Here's the drawing with two shaded views (mm, measured from the low corner). I have some questions. Give positions to 0.01 mm unless a question says otherwise; leave off trailing zeros. Loops run counter-clockwise (first coordinate to the right, second up) from the corner with the lowest first, then second, coordinate; pieces in that order, holes last.
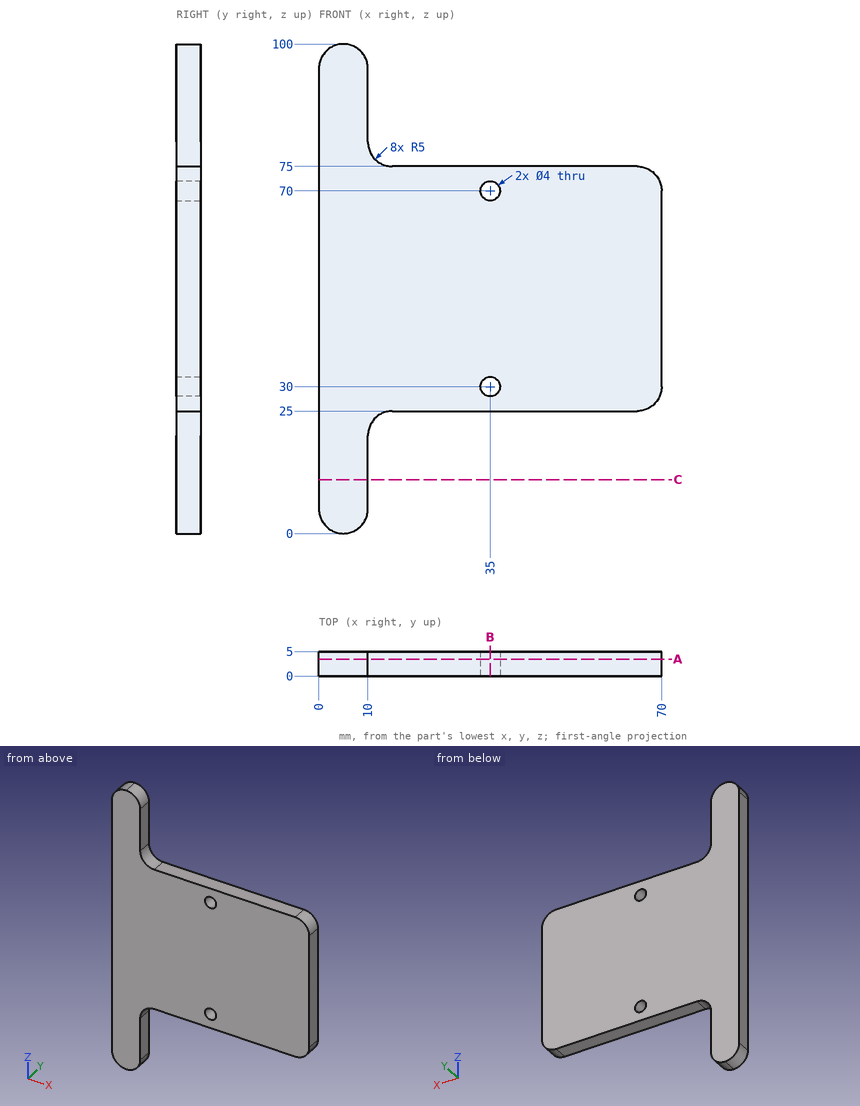
(1) Suppose I cut it at C-C on z = 11. List the corners of the cut face in (x, y) for me.
Returned:
outline: (0, 0) - (10, 0) - (10, 5) - (0, 5) - close
(2) Suppose I cut it at B-B on x = 35. List the corners of the cut face in (y, z) for me, plus the area to 3 significant figures.
Returned:
outline: (0, 25) - (5, 25) - (5, 28) - (0, 28) - close; (0, 32) - (5, 32) - (5, 68) - (0, 68) - close; (0, 72) - (5, 72) - (5, 75) - (0, 75) - close
area: 210 mm2
(3) Please list where these lines run through material, in increasing order: probe 1 along X at (y, z) = (2.7, 30); probe 2 along X at (y, z) = (3.3, 94); probe 3 along X at (y, z) = (2.55, 30.5).
Returned:
probe 1: x = 0 to 33, 37 to 70
probe 2: x = 0 to 10
probe 3: x = 0 to 33.06, 36.94 to 70
(4) Will these pins go through, and if not, where does the flat tip stop? P1, Ø1.5, axis at y = 1.5, z = 87, coming from the +X side; P2, Ø1, axis at x = 38, y = 2, coming from the +Z side.
Returned:
P1: stops at x = 10
P2: stops at z = 75
(5) Suppose I cut it at A-A on y = 3.45. Give the number of separate pieces and of enclosed holes in the cut face, plus the area to 3 significant figures.
Returned:
separate pieces: 1
enclosed holes: 2
area: 3,950 mm2
